Geometry check sheet. Reference: the model listing, model coordinates, mm. A direction names the side the tool comes from. Round coordinates to 2 decimals unless told otherwise and drop trailing zeros. Loops run counter-clockwise (first coordinate to the right, second up) from the corner with the lowest first, then second, coordinate; pieces in that order, holes last.
```python
from build123d import *

# Parameters (mm, degrees)
SKETCH1_W               = 120
SKETCH1_H               = 110
BOSS_EXTRUDE1_DEPTH     = 9
SKETCH2_W               = 9
SKETCH2_H               = 110
BOSS_EXTRUDE2_DEPTH     = 70
SKETCH3_R               = 7.5
CUT_EXTRUDE1_DEPTH      = 70
SKETCH4_R               = 3
SKETCH4_R_2             = 5
SKETCH4_R_3             = 2.5
CUT_EXTRUDE2_DEPTH      = 150.415527975
FILLET1_R               = 10
SKETCH6_R               = 3
CUT_EXTRUDE4_DEPTH      = 10
FILLET2_R               = 15
SKETCH7_W               = 45
SKETCH7_H               = 45
SKETCH7_R               = 1.65
SKETCH7_R_2             = 11.15
BOSS_EXTRUDE3_DEPTH     = 5
BOSS_EXTRUDE4_START     = -5
SKETCH8_W               = 45
SKETCH8_H               = 45
SKETCH8_R               = 1.65
SKETCH8_R_2             = 11.15
BOSS_EXTRUDE4_DEPTH     = 5
FILLET3_R               = 15
FILLET5_R               = 3
BOSS_EXTRUDE5_DEPTH     = 120
CUT_EXTRUDE5_DEPTH      = 51
CUT_EXTRUDE5_DEPTH_BACK = 10
SKETCH11_W              = 110
SKETCH11_H              = 45
FILLET6_R               = 5
FILLET7_R               = 10
BOSS_EXTRUDE6_START     = -5
BOSS_EXTRUDE6_DEPTH     = 5
BOSS_EXTRUDE7_START     = -5
BOSS_EXTRUDE7_DEPTH     = 5


# Some blends are built 0.0001 mm under size
with BuildPart() as part:
    # Sketch1 → Boss-Extrude1 (new body)
    with BuildSketch(Plane(origin=(0, 0, 0), x_dir=(1, 0, 0), z_dir=(0, 1, 0))):
        Rectangle(SKETCH1_W, SKETCH1_H)
    extrude(amount=BOSS_EXTRUDE1_DEPTH)

    # Sketch2 → Boss-Extrude2 (add)
    with BuildSketch(Plane.XZ):
        with Locations((-55.5, 0)):
            Rectangle(SKETCH2_W, SKETCH2_H)
        with Locations((55.5, 0)):
            Rectangle(SKETCH2_W, SKETCH2_H)
    extrude(amount=BOSS_EXTRUDE2_DEPTH)

    # Sketch3 → Cut-Extrude1 (cut)
    with BuildSketch(Plane.XZ):
        with Locations(Location((0, 0, 0), (0, 0, 270))):
            Circle(SKETCH3_R)
    extrude(amount=-CUT_EXTRUDE1_DEPTH, mode=Mode.SUBTRACT)

    # Sketch4 → Cut-Extrude2 (cut, through all)
    with BuildSketch(Plane.ZY.offset(60)):
        with Locations((7.875, -56.203932664)):
            Circle(SKETCH4_R)
        with Locations((26.125, -24.594005426)):
            Circle(SKETCH4_R)
        with Locations((17, -40.398969045)):
            Circle(SKETCH4_R_2)
        with Locations((-31, -22.148969045)):
            Circle(SKETCH4_R_3)
        with Locations((-31, -58.648969045)):
            Circle(SKETCH4_R_3)
        with Locations((-31, -40.398969045)):
            Circle(SKETCH4_R_2)
    extrude(amount=-CUT_EXTRUDE2_DEPTH, mode=Mode.SUBTRACT)

    # Fillet1
    fillet1_edges = [part.edges().sort_by_distance(p)[0] for p in [
        (-51, 0, 0),
        (51, 0, 0),
    ]]
    fillet(fillet1_edges, radius=FILLET1_R)

    # Sketch6 → Cut-Extrude4 (cut)
    with BuildSketch(Plane(origin=(0, 9, 0), x_dir=(1, 0, 0), z_dir=(0, 1, 0))):
        with Locations(Location((-16, 0, 0), (0, 0, 270))):
            Circle(SKETCH6_R)
        with Locations(Location((16, 0, 0), (0, 0, 270))):
            Circle(SKETCH6_R)
    extrude(amount=-CUT_EXTRUDE4_DEPTH, mode=Mode.SUBTRACT)

    # Fillet2
    fillet2_edges = [part.edges().sort_by_distance(p)[0] for p in [
        (-55.5, -70, 55),
        (55.5, -70, 55),
    ]]
    fillet(fillet2_edges, radius=FILLET2_R)

    # Sketch7 → Boss-Extrude3 (add)
    with BuildSketch(Plane(origin=(60, 0, 0), x_dir=(0, 0, -1), z_dir=(1, 0, 0))):
        with Locations((77.5, -41.5)):
            Rectangle(SKETCH7_W, SKETCH7_H)
        with Locations((63.5, -24.898969045)):
            Circle(SKETCH7_R, mode=Mode.SUBTRACT)
        with Locations((94.5, -24.898969045)):
            Circle(SKETCH7_R, mode=Mode.SUBTRACT)
        with Locations((94.5, -55.898969045)):
            Circle(SKETCH7_R, mode=Mode.SUBTRACT)
        with Locations((63.5, -55.898969045)):
            Circle(SKETCH7_R, mode=Mode.SUBTRACT)
        with Locations((79, -40.398969045)):
            Circle(SKETCH7_R_2, mode=Mode.SUBTRACT)
    extrude(amount=-BOSS_EXTRUDE3_DEPTH)

    # Sketch8 → Boss-Extrude4 (add)
    with BuildSketch(Plane.ZY.offset(60).offset(BOSS_EXTRUDE4_START)):
        with Locations((-77.5, -41.5)):
            Rectangle(SKETCH8_W, SKETCH8_H)
        with Locations(Location((-94.5, -24.898969045, 0), (0, 0, 180))):
            Circle(SKETCH8_R, mode=Mode.SUBTRACT)
        with Locations(Location((-63.5, -24.898969045, 0), (0, 0, 180))):
            Circle(SKETCH8_R, mode=Mode.SUBTRACT)
        with Locations(Location((-94.5, -55.898969045, 0), (0, 0, 180))):
            Circle(SKETCH8_R, mode=Mode.SUBTRACT)
        with Locations(Location((-63.5, -55.898969045, 0), (0, 0, 180))):
            Circle(SKETCH8_R, mode=Mode.SUBTRACT)
        with Locations(Location((-79, -40.398969045, 0), (0, 0, 180))):
            Circle(SKETCH8_R_2, mode=Mode.SUBTRACT)
    extrude(amount=BOSS_EXTRUDE4_DEPTH)

    # Fillet3
    fillet3_edges = [part.edges().sort_by_distance(p)[0] for p in [
        (57.5, -19, -55),
        (-57.5, -19, -55),
    ]]
    fillet(fillet3_edges, radius=FILLET3_R)

    # Fillet5
    fillet5_edges = [part.edges().sort_by_distance(p)[0] for p in [
        (-57.5, -64, -55),
        (-55.5, -70, -55),
        (55.5, -70, -55),
        (57.5, -64, -55),
    ]]
    fillet(fillet5_edges, radius=FILLET5_R - 0.0001)  # a hair under: the kernel refuses the full size

    # Sketch10 → Boss-Extrude5 (add)
    with BuildSketch(Plane(origin=(60, 0, 0), x_dir=(0, 0, -1), z_dir=(1, 0, 0))):
        Polygon((55, 9), (100, -19), (90.555773444, -19), (55, 3.123592365), align=None)
    extrude(amount=-BOSS_EXTRUDE5_DEPTH)

    # Sketch11 → Cut-Extrude5 (cut, two sides: drawn at the far end of the back side and taken through both)
    with BuildSketch(Plane(origin=(0, 0, 0), x_dir=(-1, 0, 0), z_dir=(0, -1, 0)).offset(-CUT_EXTRUDE5_DEPTH_BACK)):
        with Locations((0, 77.5)):
            Rectangle(SKETCH11_W, SKETCH11_H)
    extrude(amount=CUT_EXTRUDE5_DEPTH + CUT_EXTRUDE5_DEPTH_BACK, mode=Mode.SUBTRACT)

    # Fillet6
    # the kernel refuses this fillet: 5 mm, written as the material it adds along each edge
    with BuildSketch(Plane(origin=(-55, 3.123592365, -55), x_dir=(0, -1, 0), z_dir=(-1, 0, 0)), Plane(origin=(60, 3.123592365, -55), x_dir=(0, -1, 0), z_dir=(-1, 0, 0))) as fillet6_piece_1:
        with BuildLine():
            CenterArc((FILLET6_R * 1.8, -FILLET6_R), FILLET6_R, 90, 121.890791802)
            Line((FILLET6_R * 0.950943396226, -FILLET6_R * 1.52830188679), (0, 0))
            Line((0, 0), (FILLET6_R * 1.8, 0))
        make_face()
    extrude(amount=5)
    with BuildSketch(Plane(origin=(-55, -19, -90.555773444), x_dir=(0, 0.528301886792453, 0.8490566037735847), z_dir=(-1, 0, 0))) as fillet6_piece_2:
        with BuildLine():
            CenterArc((FILLET6_R * 3.5, -FILLET6_R), FILLET6_R, 90, 148.109208198)
            Line((FILLET6_R * 2.97169811321, -FILLET6_R * 1.84905660377), (0, 0))
            Line((0, 0), (FILLET6_R * 3.5, 0))
        make_face()
    extrude(amount=5)
    with BuildSketch(Plane(origin=(60, -19, -90.555773444), x_dir=(0, 0, 1), z_dir=(-1, 0, 0))) as fillet6_piece_3:
        with BuildLine():
            CenterArc((FILLET6_R * 3.5, FILLET6_R), FILLET6_R, 121.890791802, 148.109208198)
            Line((FILLET6_R * 2.97169811321, FILLET6_R * 1.84905660377), (0, 0))
            Line((0, 0), (FILLET6_R * 3.5, 0))
        make_face()
    extrude(amount=5)
    # the kernel refuses this fillet: 5 mm, written as the material it takes off along each edge
    with BuildSketch(Plane(origin=(-48.055555556, -19, -100), x_dir=(0, 0.5283018867924467, 0.8490566037735887), z_dir=(-1, 0, 0))) as fillet6_2_piece_1:
        with BuildLine():
            CenterArc((FILLET6_R * 0.555555555556, -FILLET6_R), FILLET6_R, 90, 58.109208198)
            Line((-FILLET6_R * 0.293501048218, -FILLET6_R * 0.471698113208), (0, 0))
            Line((0, 0), (FILLET6_R * 0.555555555556, 0))
        make_face()
    extrude(amount=18.888888889, mode=Mode.SUBTRACT)
    with BuildSketch(Plane(origin=(66.944444444, -19, -100), x_dir=(0, -1, 0), z_dir=(-1, 0, 0))) as fillet6_2_piece_2:
        with BuildLine():
            CenterArc((FILLET6_R * 0.555555555556, FILLET6_R), FILLET6_R, 211.890791802, 58.109208198)
            Line((-FILLET6_R * 0.293501048218, FILLET6_R * 0.471698113208), (0, 0))
            Line((0, 0), (FILLET6_R * 0.555555555556, 0))
        make_face()
    extrude(amount=18.888888889, mode=Mode.SUBTRACT)

    # Fillet7
    fillet7_edges = [part.edges().sort_by_distance(p)[0] for p in [
        (57.5, -64, -100),
        (-57.5, -64, -100),
    ]]
    fillet(fillet7_edges, radius=FILLET7_R)

    # Sketch12 → Boss-Extrude6 (add)
    with BuildSketch(Plane.ZY.offset(60).offset(BOSS_EXTRUDE6_START)):
        Polygon((-58.940723001, 2.767041623), (-81.499265811, -11.693562742), (-78.607144938, -21.141157594), (-64.532156689, -21.141157594), (-49.355143029, -12.186463132), (-49.355143029, -1.853525156), align=None)
    extrude(amount=BOSS_EXTRUDE6_DEPTH)

    # Sketch13 → Boss-Extrude7 (add)
    with BuildSketch(Plane(origin=(60, 0, 0), x_dir=(0, 0, -1), z_dir=(1, 0, 0)).offset(BOSS_EXTRUDE7_START)):
        Polygon((56.819834361, 2.885240591), (82.463306102, -10.418515425), (80.920841636, -18.902069986), (69.641570231, -22.372615034), (52.57805708, -14.660292706), (45.05854281, -6.562354261), (48.818299945, 0.68471384), (56.819834361, 0.68471384), align=None)
    extrude(amount=BOSS_EXTRUDE7_DEPTH)


solid = part.part
```
1) Sectioned sample at C-C, the plane z = 17. Record the cut outline in (x, y).
Report:
outline: (-60, -70) - (-51, -70) - (-51, -45.4) - (-60, -45.4) - close; (-60, -35.4) - (-51, -35.4) - (-51, -10) arc R10 cw to (-41, 0) - (41, 0) arc R10 cw to (51, -10) - (51, -35.4) - (60, -35.4) - (60, 9) - (-60, 9) - close; (51, -70) - (60, -70) - (60, -45.4) - (51, -45.4) - close
2) Mould release check, pull along X, two halves, no side actions. Record for faces 1 (the face through (-55.563, -53.674, 9.488)), 2 (the face through (-60, -35, -14)), 3 (the face through (-51, -40, -1)): +X half, -X half, draft (parallel to the pull), parting line (faces both ways), or undercut.
Report:
face 1: draft
face 2: -X half
face 3: undercut
3) Scan lines: line 1 along X through (y, z) = (-65, 12); line 2 along X through (y, z) = (6, 0); line 3 along X through (y, z) = (-29, -84.5). Record each from-to range of solid material in increasing order.
Report:
line 1: x = -60 to -51, 51 to 60
line 2: x = -60 to -19, -13 to -7.5, 7.5 to 13, 19 to 60
line 3: x = -60 to -55, 55 to 60
4) Gauge pin test, flat end, axial feed: pin 1 (6 mm diameter, centred on y = -33, z = -82, fed in from -X). Record the tip position at first contact, or that the pin passes through.
Report:
pin 1: passes through
5) Sectioned sample at D-D, the plane z = -31. State how many separate pieces and enclosed holes the cut face has, then the cut area to 3 significant figures.
Report:
separate pieces: 7
enclosed holes: 0
area: 2,020 mm2
6) Access from +Z, -Z, +X, -X, +Y, -Y to the whole of each face (thin tool, end or side, straight path). Record for faces 4 (the face through (55.44, -56.17, -31.33)), 5 (the face through (58, -64, -74)), 6 (the face through (13.07, 4.56, -0.65)), 7 (the face through (55, -28, -72)), 8 (the face through (-48.15, -3.01, 0.77)).
Report:
face 4: +X, -X
face 5: -Z, +X, -X, -Y
face 6: +Y, -Y
face 7: -Z, +Y, -Y
face 8: +Z, -Z, -Y
7) Sectioned sample at A-A, the plane z = 0. Record the cut outline in (x, y), then the cut area to 3 significant figures.
Report:
outline: (-60, -70) - (-51, -70) - (-51, -10) arc R10 cw to (-41, 0) - (-19, 0) - (-19, 9) - (-60, 9) - close; (-13, 0) - (-7.5, 0) - (-7.5, 9) - (-13, 9) - close; (7.5, 0) - (13, 0) - (13, 9) - (7.5, 9) - close; (19, 0) - (41, 0) arc R10 cw to (51, -10) - (51, -70) - (60, -70) - (60, 9) - (19, 9) - close
area: 2,140 mm2
8) Sectioned sample at B-B, the plane x = 0. Record the cut outline in (y, z), then the cut area to 3 significant figures.
Report:
outline: (0, -55) - (9, -55) - (9, -7.5) - (0, -7.5) - close; (0, 7.5) - (9, 7.5) - (9, 55) - (0, 55) - close
area: 855 mm2
